from build123d import *

# Parameters (mm, degrees)
F0_R     = 1.5
F0_W     = 65
F0_H     = 59.651572
F1_DEPTH = 5


with BuildPart() as f1:
    # F0 (on Top) → F1 (new body)
    with BuildSketch(Plane.XY):
        with BuildLine():
            Line((5.892689, 0), (-59.107311, 0))
            Line((-59.107311, 0), (-59.107311, -60.348428))
            Line((-59.107311, -60.348428), (5.892689, -60.348428))
            Line((5.892689, -60.348428), (5.892689, -50.649721))
            ThreePointArc((5.892689, -50.649721), (-9.211324, -35.650082), (5.892689, -20.650443))
            Line((5.892689, -20.650443), (5.892689, -18.074285))
            ThreePointArc((5.892689, -18.074285), (4.891486, -16.659647), (5.892689, -15.245008))
            Line((5.892689, -15.245008), (5.892689, 0))
        make_face()
        with Locations((-10.958927, -44.623251)):
            Circle(F0_R, mode=Mode.SUBTRACT)
        with Locations((-26.607311, 29.825786)):
            Rectangle(F0_W, F0_H)
        with Locations((-48.146435, 25.644738)):
            Circle(F0_R, mode=Mode.SUBTRACT)
        with Locations((-42.146435, 25.644738)):
            Circle(F0_R, mode=Mode.SUBTRACT)
        with Locations((-36.146435, 25.644738)):
            Circle(F0_R, mode=Mode.SUBTRACT)
        with Locations((-48.146435, 54.644738)):
            Circle(F0_R, mode=Mode.SUBTRACT)
        with Locations((-42.146435, 54.644738)):
            Circle(F0_R, mode=Mode.SUBTRACT)
        with Locations((-36.146435, 54.644738)):
            Circle(F0_R, mode=Mode.SUBTRACT)
        with Locations((38.392689, 29.825786)):
            Rectangle(F0_W, F0_H)
        with Locations((47.931814, 25.644738)):
            Circle(F0_R, mode=Mode.SUBTRACT)
        with Locations((53.931814, 25.644738)):
            Circle(F0_R, mode=Mode.SUBTRACT)
        with Locations((59.931814, 25.644738)):
            Circle(F0_R, mode=Mode.SUBTRACT)
        with Locations((47.931814, 54.644738)):
            Circle(F0_R, mode=Mode.SUBTRACT)
        with Locations((53.931814, 54.644738)):
            Circle(F0_R, mode=Mode.SUBTRACT)
        with Locations((59.931814, 54.644738)):
            Circle(F0_R, mode=Mode.SUBTRACT)
        with BuildLine():
            Line((70.892689, 0), (5.892689, 0))
            Line((5.892689, 0), (5.892689, -15.245008))
            ThreePointArc((5.892689, -15.245008), (7.258032, -15.435271), (7.891486, -16.659647))
            ThreePointArc((7.891486, -16.659647), (7.258032, -17.884023), (5.892689, -18.074285))
            Line((5.892689, -18.074285), (5.892689, -20.650443))
            ThreePointArc((5.892689, -20.650443), (16.431989, -25.080318), (20.788676, -35.650082))
            ThreePointArc((20.788676, -35.650082), (16.431989, -46.219846), (5.892689, -50.649721))
            Line((5.892689, -50.649721), (5.892689, -60.348428))
            Line((5.892689, -60.348428), (70.892689, -60.348428))
            Line((70.892689, -60.348428), (70.892689, 0))
        make_face()
        with Locations((21.933471, -45.667347)):
            Circle(F0_R, mode=Mode.SUBTRACT)
    extrude(amount=F1_DEPTH)


solid = f1.part
Source: CAD feature listing. Evaluate the final solid. Frame: model axes, mm. Coordinates: 2 decimals unless noted, no trailing zeros. Loops run counter-clockwise (first coordinate to the right, second up) from the corner with the lowest first, then second, coordinate; pieces in that order, holes last. Notation, with made-up numbers: (58, 21.5) - (86, 21.5) arc R27 cw to (86, 44.5) - close; hole circle Ø10 at (45.25, -6). An arc over 180 degrees is marked (long way). Return JSON: item names as keys, results as strings.
Q1. Section C-C, the plane z = 0.9. Give the number of separate pieces and of enclosed holes in the cut face, plus the area to 3 significant figures.
Results:
{"separate pieces": "1", "enclosed holes": "16", "area": "14,800 mm2"}
Q2. Section B-B, the plane x = -5. Return loops of the section in (y, z), plus the area to 3 significant figures.
Results:
{"outline": "(-60.35, 0) - (-46.07, 0) - (-46.07, 5) - (-60.35, 5) - close; (-25.23, 0) - (59.65, 0) - (59.65, 5) - (-25.23, 5) - close", "area": "496 mm2"}
Q3. Section A-A, the plane y = -34. Return loops of the section in (x, z), plus the area to 3 significant figures.
Results:
{"outline": "(-59.11, 0) - (-9.12, 0) - (-9.12, 5) - (-59.11, 5) - close; (20.7, 0) - (70.89, 0) - (70.89, 5) - (20.7, 5) - close", "area": "501 mm2"}
Q4. Contact query for a flat-ended pin moving along its axis: P1, Ø2.5, axis at x = 21.93, y = -45.67, coming from the +Z side. Output: stop coordinate, or through.
Results:
{"P1": "through"}
Q5. Material intervals for line 1 along Y through (x, z) = (-48, 0.35); line 2 along Y through (x, z) = (53, 2); line 3 along Y through (x, z) = (10.5, 3.15), sorted ascending.
Results:
{"line 1": "-60.35 to 24.15, 27.14 to 53.15, 56.14 to 59.65", "line 2": "-60.35 to 24.47, 26.82 to 53.47, 55.82 to 59.65", "line 3": "-60.35 to -49.89, -21.41 to 59.65"}
Q6. Mould query, pull axis Y, two halves, no side actions, for faces 1 (the flat face through (7, 59.652, 2)), 2 (the cylindrical face through (-37.645, 25.711, 2.465)), 3 (the flat face through (-59.107, 0, 2)). Classes: released by +Y, released by -Y, zero draft, split by the parting line, or undercut.
Results:
{"face 1": "released by +Y", "face 2": "undercut", "face 3": "zero draft"}
